Geometry: final body of the model. Coordinates: model frame, mm. Face numbers are marked on the shaded views. A direction names the side the tool comes from. Give positions to 0.01 mm unless a question says otherwise; leave off trailing zeros. Order: outer loops, then holes, each group sorted by start corner. A loop starts at its lowest first (then second) coordinate and runs counter-clockwise, first axis right, second up. Notation, with made-up numbers: (3.25, 57.25) -> (35.25, 57.25) arc R28 cw to (35.25, 88.25) -> close; hole circle Ø7 at (61, 55.25). An arc over 180 degrees is marked (long way). Write item = value, one per line.
```python
from build123d import *

# Parameters (mm, degrees)
F0_W      = 42
F0_H      = 42
F0_R      = 1.75
F0_R_2    = 12
F1_DEPTH  = 7
F0_W_2    = 3
F2_DEPTH  = 45
F3_DEPTH  = 45
F4_SIZE2  = 38
F4_SIZE   = 42
F5_R      = 2.25
F6_DEPTH  = 25
F7_R      = 5
F8_R      = 2.99999
F9_W      = 26
F9_H      = 22
F10_DEPTH = 25
F11_R     = 5


# Not quite as in the source:
# - a fillet or chamfer is up to 0.001 mm smaller than in the source, because OpenCascade refuses the exact size


with BuildPart() as f1:
    # F0 (on Front) → F1 (new body)
    with BuildSketch(Plane.XZ):
        Rectangle(F0_W, F0_H)
        with Locations((-15.5, -15.5)):
            Circle(F0_R, mode=Mode.SUBTRACT)
        with Locations((15.5, -15.5)):
            Circle(F0_R, mode=Mode.SUBTRACT)
        with Locations((-15.5, 15.5)):
            Circle(F0_R, mode=Mode.SUBTRACT)
        Circle(F0_R_2, mode=Mode.SUBTRACT)
        with Locations((15.5, 15.5)):
            Circle(F0_R, mode=Mode.SUBTRACT)
    extrude(amount=-F1_DEPTH)

    # F0 (on Front) → F2 (join)
    with BuildSketch(Plane.XZ):
        with Locations((22.5, 0)):
            Rectangle(F0_W_2, F0_H)
        with Locations((-22.5, 0)):
            Rectangle(F0_W_2, F0_H)
    extrude(amount=-F2_DEPTH)

    # F0 (on Front) → F3 (join, through all)
    with BuildSketch(Plane.XZ):
        Polygon((24, -21), (21, -21), (-21, -21), (-24, -21), (-32, -21), (-32, -25), (32, -25), (32, -21), align=None)
    extrude(amount=-F3_DEPTH)

    # F4
    f4_edges = [f1.edges().sort_by_distance(p)[0] for p in [
        (22.5, 45, 21),
        (-22.5, 45, 21),
    ]]
    f4_side = f1.faces().sort_by_distance((-31.211838, 45, -23))[0]
    chamfer(f4_edges, length=F4_SIZE, length2=F4_SIZE2, reference=f4_side)

    # F5 (on face) → F6 (cut)
    with BuildSketch(Plane.XY.offset(-21)):
        with Locations((28, 7.5)):
            Circle(F5_R)
        with Locations((28, 22.5)):
            Circle(F5_R)
        with Locations((28, 37.5)):
            Circle(F5_R)
        with Locations((-28, 7.5)):
            Circle(F5_R)
        with Locations((-28, 22.5)):
            Circle(F5_R)
        with Locations((-28, 37.5)):
            Circle(F5_R)
    extrude(amount=-F6_DEPTH, mode=Mode.SUBTRACT)

    # F7
    f7_edges = [f1.edges().sort_by_distance(p)[0] for p in [
        (-32, 0, -23),
        (-32, 45, -23),
        (32, 0, -23),
        (32, 45, -23),
    ]]
    fillet(f7_edges, radius=F7_R)

    # F8 (radius 3 in the source; OpenCascade refuses exactly that, so slightly less here)
    f8_edges = [f1.edges().sort_by_distance(p)[0] for p in [
        (24, 0, 0),
        (-24, 0, 0),
        (-24, 26, 0),
        (-24, 3.5, 21),
        (24, 3.5, 21),
        (24, 26, 0),
    ]]
    fillet(f8_edges, radius=F8_R)

    # F9 (on face) → F10 (cut)
    with BuildSketch(Plane.XY.offset(-21)):
        with Locations((0, 26)):
            Rectangle(F9_W, F9_H)
    extrude(amount=-F10_DEPTH, mode=Mode.SUBTRACT)

    # F11
    f11_edges = [f1.edges().sort_by_distance(p)[0] for p in [
        (13, 15, -23),
        (-13, 15, -23),
        (-13, 37, -23),
        (13, 37, -23),
    ]]
    fillet(f11_edges, radius=F11_R)


solid = f1.part
```
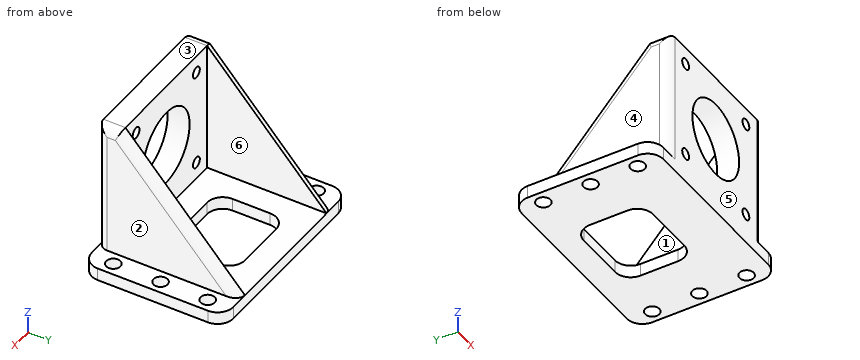
1) Section query B-B (x = 28). Output: boundary loops of the cut face in (y, z), plus the area to 3 significant figures.
Check sheet entries:
outline = (0.1, -25) -> (5.25, -25) -> (5.25, -21) -> (0.1, -21) -> close; (9.75, -25) -> (20.25, -25) -> (20.25, -21) -> (9.75, -21) -> close; (24.75, -25) -> (35.25, -25) -> (35.25, -21) -> (24.75, -21) -> close; (39.75, -25) -> (44.9, -25) -> (44.9, -21) -> (39.75, -21) -> close
area = 125 mm²
2) Line query: line 1 (Y direction, x = -28, z = -23); line 2 (X direction, y = 7, z = -22); line 3 (X direction, y = 16.5, z = -20.5). Output: solid intervals per line, ascending. Write a range as from..to.
Check sheet entries:
line_1 = 0.1..5.25, 9.75..20.25, 24.75..35.25, 39.75..44.9
line_2 = -32..-30.19, -25.81..25.81, 30.19..32
line_3 = -24..-21, 21..24
3) Section query D-D (x = -15.5). Output: boundary loops of the cut face in (y, z), plus the area to 3 significant figures.
Check sheet entries:
outline = (0, -25) -> (45, -25) -> (45, -21) -> (7, -21) -> (7, -17.25) -> (0, -17.25) -> close; (0, -13.75) -> (7, -13.75) -> (7, 13.75) -> (0, 13.75) -> close; (0, 17.25) -> (7, 17.25) -> (7, 21) -> (0, 21) -> close
area = 425 mm²
4) Mould query, pull axis X, two halves, no side actions, for the marked faces 1, 2, 3 and 4. Classes: +X half, -X half, draft (parallel to the pull), parting line (faces both ways), or undercut.
Check sheet entries:
face_1 = undercut
face_2 = +X half
face_3 = draft
face_4 = -X half
5) First-contact query: P1, Ø4, axis at x = -15.5, z = -15.5, coming from the -Y side; P2, Ø6, axis at y = 15, z = -14, coming from the -X side; P3, Ø10, axis at x = 12.5, z = 3, coming from the +Y side; P4, Ø12, axis at y = 15, z = 12.5, coming from the +X side. Flat tips, straight axial feed; report the tip coordinate or a pass-through.
Check sheet entries:
P1 = 0
P2 = -24
P3 = 7
P4 = 24
6) Section query C-C (y = 4). Output: boundary loops of the cut face in (x, z).
Check sheet entries:
outline = (-31.9, -25) -> (31.9, -25) -> (31.9, -21) -> (24, -21) -> (24, 18) arc R3 ccw to (21, 21) -> (-21, 21) arc R3 ccw to (-24, 18) -> (-24, -21) -> (-31.9, -21) -> close; hole circle Ø3.5 at (-15.5, -15.5); hole circle Ø3.5 at (-15.5, 15.5); hole circle Ø24 at (0, 0); hole circle Ø3.5 at (15.5, -15.5); hole circle Ø3.5 at (15.5, 15.5)
7) Reachability of the marked faces 5 and 6 from +Z, -Z, +X, -X, +Y, -Y: full face, straight path, thin tool, end or side. Return the list, or none.
Check sheet entries:
face_5 = +Z, -Z, +X, -X, -Y
face_6 = +Z, +Y
8) Section query A-A (x = 0). Output: boundary loops of the cut face in (y, z), plus the area to 3 significant figures.
Check sheet entries:
outline = (0, -25) -> (15, -25) -> (15, -21) -> (7, -21) -> (7, -12) -> (0, -12) -> close; (0, 12) -> (7, 12) -> (7, 21) -> (0, 21) -> close; (37, -25) -> (45, -25) -> (45, -21) -> (37, -21) -> close
area = 218 mm²
